Could you check a few things on this model? Use its own coordinates, in mm. Face numbers are marked on the shaded views. Round coordinates to 2 decimals unless told otherwise and drop trailing zeros. Write each loop counter-clockwise with the first axis right and the second up, starting at its lowest first coordinate (ties: lowest second). Pieces come first, ordered by that corner, then holes. Notation, with made-up numbers: (87.5, -3) - (111.5, -3) arc R31 cw to (111.5, 36) - close; hole circle Ø4 at (-15, 74.5). An arc over 180 degrees is marked (long way). Write each question's results on one line, items separated by ' | '. Start each with the question number.
(1) Imagine slicing it at A-A on y = 39. Write out the boundary of the cut face in (x, z).
(2) For P1, Ø1.5, axis at y = 35.5, z = 2.5, coming from the -X side; P2, Ø1.5, axis at x = 4, y = 41.5, coming from the +Z side, each with a flat end and sliding along its axis, tell me the tip position at first contact or that it passes through.
(3) Imagine slicing it at C-C on z = 0.8. Write out the boundary of the cut face in (x, y).
(4) Thinking about a two-plate mould opening in X: for the marked faces 1 and 2, which applies, +X half, -X half, draft (parallel to the pull), parting line (faces both ways), or undercut?
(5) Imagine slicing it at B-B on x = 4. Write out the boundary of the cut face in (y, z), then the cut area to 3 significant figures.
(6) Please list where these lines run through material, in increasing order: line 1 (X direction, y = 42, z = 2.25); line 2 (Z direction, x = 26.5, y = 40.5); line 3 (X direction, y = 5, z = 2.25). Write a range as [from, to].
(7) Imagine slicing it at D-D on x = 24. Write out the boundary of the cut face in (y, z).
```python
from build123d import *

# Parameters (mm, degrees)
PAD_DEPTH    = 3
POCKET_DEPTH = 1


with BuildPart() as part:
    # Sketch → Pad (new body)
    with BuildSketch(Plane.XY):
        with BuildLine():
            Line((0, 0), (8, 0))
            ThreePointArc((8, 0), (24.970563, 7.029437), (32, 24))
            Line((32, 24), (32, 83))
            Line((32, 83), (0, 83))
            Line((0, 83), (0, 0))
        make_face()
    extrude(amount=PAD_DEPTH)

    # Sketch001 (on Face7 of Pad) → Pocket (cut)
    with BuildSketch(Plane.XY.offset(3)):
        with BuildLine():
            Line((3, 84), (3, 3))
            Line((3, 3), (8, 3))
            ThreePointArc((8, 3), (22.849242, 9.150758), (29, 24))
            Line((29, 24), (29, 84))
            Line((29, 84), (3, 84))
        make_face()
    extrude(amount=-POCKET_DEPTH, mode=Mode.SUBTRACT)


solid = part.part
```
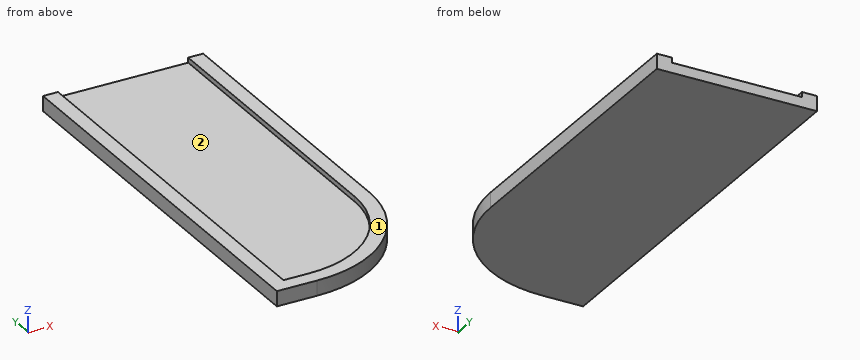
Response:
1) outline: (0, 0) - (32, 0) - (32, 3) - (29, 3) - (29, 2) - (3, 2) - (3, 3) - (0, 3) - close
2) P1: x = 0 | P2: z = 2
3) outline: (0, 0) - (8, 0) arc R24 ccw to (32, 24) - (32, 83) - (0, 83) - close
4) face 1: draft | face 2: undercut
5) outline: (0, 0) - (83, 0) - (83, 2) - (3, 2) - (3, 3) - (0, 3) - close | area: 169 mm²
6) line 1: [0, 3], [29, 32] | line 2: [0, 2] | line 3: [0, 3], [16.94, 22.66]
7) outline: (6.11, 0) - (83, 0) - (83, 2) - (10.4, 2) - (10.4, 3) - (6.11, 3) - close
